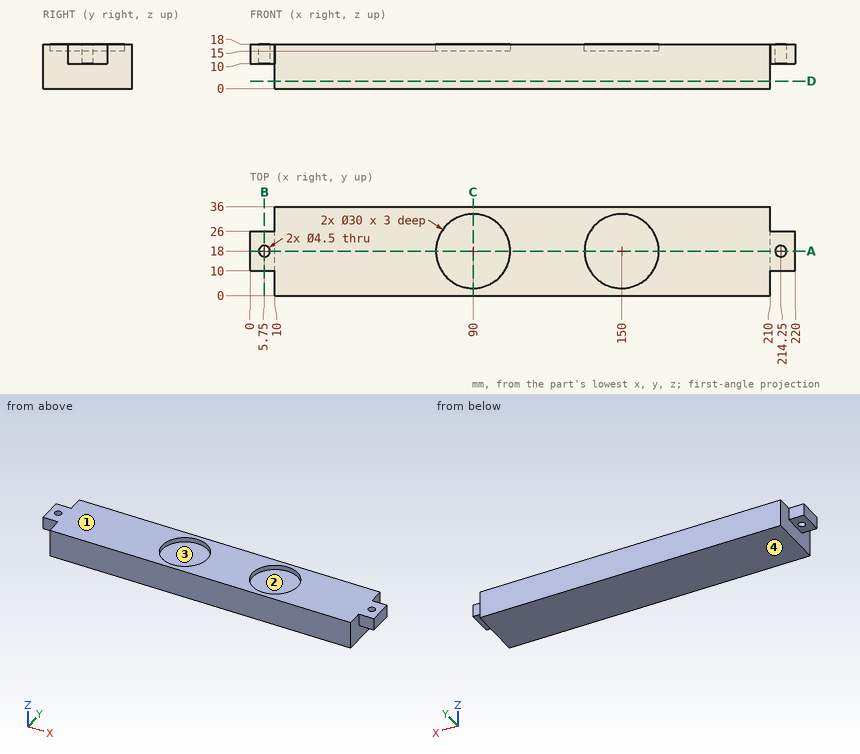
Answer from the drawing. Dimensions are ordinates in mm from the lowest x, y and z of the part. A direction names the side the tool comes from. Round coordinates to 2 decimals unless told otherwise and drop trailing zeros. Write each loop counter-clockwise with the first axis right and the second up, starting at its lowest first coordinate (ties: lowest second). Pieces come first, ordered by that corner, then holes. Notation, with made-up numbers: (85.5, -3) - (139.5, -3) arc R33 ccw to (139.5, 30) - close; hole circle Ø9 at (-21.5, 5). An arc over 180 degrees is marked (long way). One line per item, written item: value.
Q1. Find section D-D (z = 3). Determine the outline of the cut face in (x, y).
The answers:
outline: (10, 0) - (210, 0) - (210, 36) - (10, 36) - close
Q2. Straight lines are drawn through the part: line 1 (Y direction, x = 150, z = 15.9); line 2 (Y direction, x = 5.75, z = 13.75); line 3 (X direction, y = 16, z = 14.25). For each, find the intervals that lie inside material, in ascending order. Write a range as from..to.
The answers:
line 1: y = 0..3, 33..36
line 2: y = 10..15.75, 20.25..26
line 3: x = 0..4.72, 6.78..213.22, 215.28..220
Q3. For a pull along X with two mould halves and no side action, classify the marked faces 1 and 2 as pulls with the +X half, pulls with the -X half, needs draft (parallel to the pull), parting line crosses it, or undercut.
The answers:
face 1: needs draft
face 2: undercut
Q4. Which of the six approach directions +Z, -Z, +X, -X, +Y, -Y give full straight-line access (tool end or side, diameter ignored) to the marked faces 3 and 4?
The answers:
face 3: +Z
face 4: -Z, +X, -X, +Y, -Y
Q5. Find section C-C (x = 90). Determine the outline of the cut face in (y, z), and give its area (3 significant figures).
The answers:
outline: (0, 0) - (36, 0) - (36, 18) - (33, 18) - (33, 15) - (3, 15) - (3, 18) - (0, 18) - close
area: 558 mm2
Q6. Each of these flat-tipped pins is pushed along its axis until it touches: P1, Ø11, axis at x = 215, y = 14, coming from the -Z side; P2, Ø2, axis at y = 8.5, z = 9, coming from the +X side; P3, Ø3, axis at y = 27.5, z = 9.5, coming from the -X side; P4, Ø2.5, axis at x = 7.5, z = 13, coming from the -Y side. Where does it stop, or does it pass through?
The answers:
P1: stops at z = 0
P2: stops at x = 210
P3: stops at x = 10
P4: stops at y = 10
Q7. Find section B-B (x = 5.75). Determine the outline of the cut face in (y, z), and give its area (3 significant figures).
The answers:
outline: (10, 10) - (15.75, 10) - (15.75, 18) - (10, 18) - close; (20.25, 10) - (26, 10) - (26, 18) - (20.25, 18) - close
area: 92.0 mm2
Q8. Find section A-A (y = 18). Determine the outline of the cut face in (x, z), and give its area (3 significant figures).
The answers:
outline: (0, 10) - (3.5, 10) - (3.5, 18) - (0, 18) - close; (8, 10) - (10, 10) - (10, 0) - (210, 0) - (210, 10) - (212, 10) - (212, 18) - (165, 18) - (165, 15) - (135, 15) - (135, 18) - (105, 18) - (105, 15) - (75, 15) - (75, 18) - (8, 18) - close; (216.5, 10) - (220, 10) - (220, 18) - (216.5, 18) - close
area: 3,510 mm2
